For this review, take the finished solid that the model builds, in its own axes (mm). Face numbers are marked on the shaded views. A direction names the side the tool comes from. Coordinates: 2 decimals unless noted, no trailing zeros. Loops run counter-clockwise (first coordinate to the right, second up) from the corner with the lowest first, then second, coordinate; pieces in that order, holes last. Notation, with made-up numbers: M -36.5,43 L -15.5,43 A26 ccw -15.5,67 Z; hole C -39.75,32 d6. An arc over 180 degrees is marked long. Put each result on its own line as item: value.
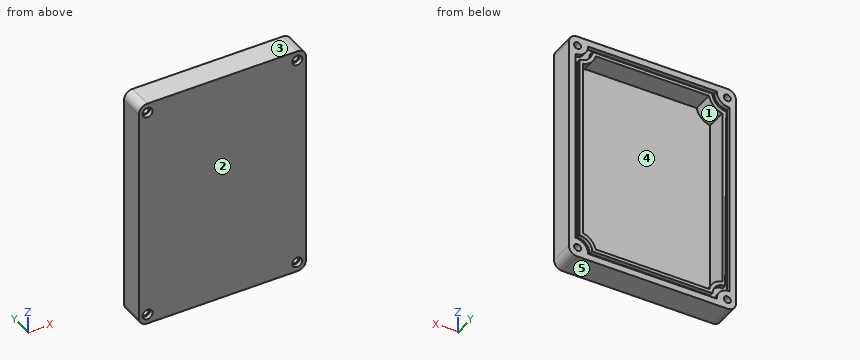
```python
from build123d import *

# Parameters (mm, degrees)
BASE_W              = 100
BASE_H              = 140
BOTTOM_DEPTH        = 2.5
WALL_W              = 100
WALL_H              = 140
WALL_W_2            = 92
WALL_H_2            = 132
WALLS_DEPTH         = 12.5
MAINFILLET_R        = 5
DRILLHOLES_R        = 2.1
DRILLING_DEPTH      = 45
SKETCH8_R           = 3
CUT_EXTRUDE2_DEPTH  = 2.5
BOSS_EXTRUDE1_DEPTH = 12.5
BOSS_EXTRUDE2_DEPTH = 10


with BuildPart() as part:
    # Base → Bottom (new body)
    with BuildSketch(Plane(origin=(0, 0, 0), x_dir=(1, 0, 0), z_dir=(0, 1, 0))):
        Rectangle(BASE_W, BASE_H)
    extrude(amount=-BOTTOM_DEPTH)

    # Wall → Walls (add)
    with BuildSketch(Plane(origin=(0, 0, 0), x_dir=(1, 0, 0), z_dir=(0, 1, 0))):
        Rectangle(WALL_W, WALL_H)
        Rectangle(WALL_W_2, WALL_H_2, mode=Mode.SUBTRACT)
        with BuildLine():
            Line((-46, -58.5), (-46, -66))
            Line((-46, -66), (-38.5, -66))
            ThreePointArc((-38.5, -66), (-40.696699141, -60.696699141), (-46, -58.5))
        make_face()
        with BuildLine():
            ThreePointArc((46, -58.5), (40.696699141, -60.696699141), (38.5, -66))
            Line((38.5, -66), (46, -66))
            Line((46, -66), (46, -58.5))
        make_face()
        with BuildLine():
            Line((-46, 66), (-46, 58.5))
            ThreePointArc((-46, 58.5), (-40.696699141, 60.696699141), (-38.5, 66))
            Line((-38.5, 66), (-46, 66))
        make_face()
        with BuildLine():
            Line((46, 66), (38.5, 66))
            ThreePointArc((38.5, 66), (40.696699141, 60.696699141), (46, 58.5))
            Line((46, 58.5), (46, 66))
        make_face()
    extrude(amount=WALLS_DEPTH)

    # MainFillet
    mainfillet_edges = [part.edges().sort_by_distance(p)[0] for p in [
        (50, 5, -70),
        (50, 5, 70),
        (-50, 5, 70),
        (-50, 5, -70),
    ]]
    fillet(mainfillet_edges, radius=MAINFILLET_R)

    # DrillHoles → Drilling (cut)
    with BuildSketch(Plane(origin=(0, 12.5, 0), x_dir=(-1, 0, 0), z_dir=(0, -1, 0))):
        with Locations((44.79923541, 64.27716385)):
            Circle(DRILLHOLES_R)
        with Locations((44.79923541, -64.27716385)):
            Circle(DRILLHOLES_R)
        with Locations((-44.79923541, -64.27716385)):
            Circle(DRILLHOLES_R)
        with Locations((-44.79923541, 64.27716385)):
            Circle(DRILLHOLES_R)
    extrude(amount=DRILLING_DEPTH, mode=Mode.SUBTRACT)

    # Sketch8 → Cut-Extrude2 (cut)
    with BuildSketch(Plane(origin=(0, -2.5, 0), x_dir=(1, 0, 0), z_dir=(0, 1, 0))):
        with Locations((-44.79923541, 64.27716385)):
            Circle(SKETCH8_R)
        with Locations((44.79923541, 64.27716385)):
            Circle(SKETCH8_R)
        with Locations((-44.79923541, -64.27716385)):
            Circle(SKETCH8_R)
        with Locations((44.79923541, -64.27716385)):
            Circle(SKETCH8_R)
    extrude(amount=CUT_EXTRUDE2_DEPTH, mode=Mode.SUBTRACT)

    # Extrusion → Boss-Extrude1 (add)
    with BuildSketch(Plane(origin=(0, 12.5, 0), x_dir=(-1, 0, 0), z_dir=(0, -1, 0))):
        with BuildLine():
            Line((44.208318845, -55.242571154), (43.54473793, 56.000133433))
            ThreePointArc((43.54473793, 56.000133433), (38.212540046, 58.180905412), (36, 63.5))
            Line((36, 63.5), (-36, 63.5))
            ThreePointArc((-36, 63.5), (-38.196699141, 58.196699141), (-43.5, 56))
            Line((-43.5, 56), (-43.5, -56))
            ThreePointArc((-43.5, -56), (-38.196699141, -58.196699141), (-36, -63.5))
            Line((-36, -63.5), (36, -63.5))
            ThreePointArc((36, -63.5), (38.401198888, -57.678453182), (44.208318845, -55.242571154))
        make_face()
        with BuildLine():
            Line((41.876528387, 53.928461988), (41.876528387, -53.242571154))
            ThreePointArc((41.876528387, -53.242571154), (36.675168704, -56.193062448), (33.919092643, -61.5))
            Line((33.919092643, -61.5), (-34, -61.5))
            ThreePointArc((-34, -61.5), (-36.635234891, -56.635234891), (-41.5, -54))
            Line((-41.5, -54), (-41.5, 54))
            ThreePointArc((-41.5, 54), (-36.635234891, 56.635234891), (-34, 61.5))
            Line((-34, 61.5), (34, 61.5))
            ThreePointArc((34, 61.5), (36.772076684, 56.501068092), (41.876528387, 53.928461988))
        make_face(mode=Mode.SUBTRACT)
    extrude(amount=BOSS_EXTRUDE1_DEPTH)

    # Gasket → Boss-Extrude2 (add)
    with BuildSketch(Plane(origin=(0, 0, 0), x_dir=(1, 0, 0), z_dir=(0, 1, 0))):
        with BuildLine():
            Line((-38.5, 66), (38.5, 66))
            ThreePointArc((38.5, 66), (40.696699141, 60.696699141), (46, 58.5))
            Line((46, 58.5), (46, -58.5))
            ThreePointArc((46, -58.5), (40.696699141, -60.696699141), (38.5, -66))
            Line((38.5, -66), (-38.5, -66))
            ThreePointArc((-38.5, -66), (-40.696699141, -60.696699141), (-46, -58.5))
            Line((-46, -58.5), (-46, 58.5))
            ThreePointArc((-46, 58.5), (-40.696699141, 60.696699141), (-38.5, 66))
        make_face()
        with BuildLine():
            Line((-36, -63.5), (36, -63.5))
            ThreePointArc((36, -63.5), (38.196699141, -58.196699141), (43.5, -56))
            Line((43.5, -56), (43.5, 56))
            ThreePointArc((43.5, 56), (38.196699141, 58.196699141), (36, 63.5))
            Line((36, 63.5), (-36, 63.5))
            ThreePointArc((-36, 63.5), (-38.212540046, 58.180905412), (-43.54473793, 56.000133433))
            Line((-43.54473793, 56.000133433), (-44.208318845, -55.242571154))
            ThreePointArc((-44.208318845, -55.242571154), (-38.401198888, -57.678453182), (-36, -63.5))
        make_face(mode=Mode.SUBTRACT)
    extrude(amount=BOSS_EXTRUDE2_DEPTH)


solid = part.part
```
(1) Tool access review of the marked faces 4 and 5: name each direction out of +Z, -Z, +X, -X, +Y, -Y from which nothing blocks a thin tool from reaching the whole face with its end or side.
Determined:
face 4: +Y
face 5: -Z, +X, -X, +Y, -Y
(2) For pin 1 (2 mm diameter, centred on x = 32.5, z = -18, fed in from +Y), flat-tipped, find the tip position at first contact; note if it passes through.
Determined:
pin 1: stops at y = 0
(3) Add section B-B (x = -23). Write out the cut boundary in (y, z).
Determined:
outline: M -2.5,-70 L 12.5,-70 L 12.5,-66 L 10,-66 L 10,-63.5 L 12.5,-63.5 L 12.5,-61.5 L 0,-61.5 L 0,61.5 L 12.5,61.5 L 12.5,63.5 L 10,63.5 L 10,66 L 12.5,66 L 12.5,70 L -2.5,70 Z
(4) Add section C-C (z = 30). Write out the cut boundary in (x, y).
Determined:
outline: M -50,-2.5 L 50,-2.5 L 50,12.5 L 46,12.5 L 46,10 L 43.5,10 L 43.5,12.5 L 41.5,12.5 L 41.5,0 L -41.88,0 L -41.88,12.5 L -44.06,12.5 L -44.06,10 L -46,10 L -46,12.5 L -50,12.5 Z
(5) Add section A-A (y = 7.5). Write out the cut boundary in (x, z), plus the area to 3 significant figures.
Determined:
outline: M -50,-65 A5 ccw -45,-70 L 45,-70 A5 ccw 50,-65 L 50,65 A5 ccw 45,70 L -45,70 A5 ccw -50,65 Z; hole C -44.8,-64.28 d4.2; hole C -44.8,64.28 d4.2; hole M -41.88,-53.93 A9.71 cw -34,-61.5 L 34,-61.5 A9.71 cw 41.5,-54 L 41.5,54 A9.71 cw 34,61.5 L -33.92,61.5 A10.53 cw -41.88,53.24 Z; hole C 44.8,-64.28 d4.2; hole C 44.8,64.28 d4.2
area: 3,840 mm^2
(6) Wall thickness on line 1 along Z through (x, y) = (-27.5, 10.5); line 2 along X through (y, z) = (8.5, -47); line 3 along Z through (x, y) = (-9.5, 6.25): over which ranges is each line inside the solid? List them lowest first. Write a range as [from, to].
Determined:
line 1: z = [-70, -66], [-63.5, -61.5], [61.5, 63.5], [66, 70]
line 2: x = [-50, -41.88], [41.5, 50]
line 3: z = [-70, -61.5], [61.5, 70]
(7) Draft analysis for pull direction Z (two halves, no side actions). For the marked faces 1, 2 and 3, state which applies: +Z half, -Z half, draft (parallel to the pull), parting line (faces both ways), or undercut.
Determined:
face 1: undercut
face 2: draft
face 3: +Z half
